Verification items for the finished model (mm, model axes). Face numbers are marked on the shaded views. Round coordinates to 2 decimals unless told otherwise and drop trailing zeros. Order: outer loops, then holes, each group sorted by start corner. A loop starts at its lowest first (then second) coordinate and runs counter-clockwise, first axis right, second up. Notation, with made-up numbers: M 66,32.5 L 121,32.5 A25 cw 121,46.5 Z; hole C -17,53.25 d1. An arc over 180 degrees is marked long. Use one line per item in the form item = value. Start each with the question number.
Item 1: Cross-section at B-B on x = -2.5. Count the separate pieces of the cut face and the enclosed holes in it, then the cut area to 3 significant figures.
Item 2: Go/stop test with a flat-tipped pin: pin 1 Ø2.5 at (y, z) = (-3.24, 4) entering from +X. Record where the tip stops, or that it passes through.
Item 3: Cross-section at A-A on z = 4. Enter the section's corners in (x, y), then the cut area to 3 significant figures.
Item 4: Thickness scan on probe 1 along Y at (x, z) = (3.25, 4); probe 2 along Y at (x, z) = (-6.5, 6.75); probe 3 along Y at (x, z) = (-1.75, 4). Record the ranges inside material, lowest first. Write a range as [from, to].
Item 5: Release check for a two-part mould opening along Y. For the marked faces 1, 2 and 3 record: +Y half, -Y half, draft (parallel to the pull), parting line (faces both ways), or undercut.
from build123d import *

# Parameters (mm, degrees)
EXTRUDE_1_DEPTH     = 8
SKETCH_2_R          = 1.7
CUT_EXTRUDE_2_DEPTH = 15
SKETCH_3_R          = 1.7
CUT_EXTRUDE_4_DEPTH = 15
CHAMFER_1_SIZE      = 0.5
SKETCH_4_R          = 1.7
CUT_EXTRUDE_5_DEPTH = 10


with BuildPart() as part:
    # 草图1 → 凸台-拉伸1 (new body)
    with BuildSketch(Plane.XY):
        with BuildLine():
            Line((-6.780789716, 23.005235362), (-6.780789716, 15.505235362))
            ThreePointArc((-6.780789716, 15.505235362), (0.719210284, 8.005235362), (-6.780789716, 0.505235362))
            Line((-6.780789716, 0.505235362), (-6.780789716, -6.994764638))
            ThreePointArc((-6.780789716, -6.994764638), (-0.358173427, -5.55020635), (4.82739705, -1.494764638))
            Line((4.82739705, -1.494764638), (4.82739705, 17.505235362))
            ThreePointArc((4.82739705, 17.505235362), (-0.358173427, 21.560677073), (-6.780789716, 23.005235362))
        make_face()
    extrude(amount=EXTRUDE_1_DEPTH)

    # 草图2 → 切除-拉伸2 (cut)
    with BuildSketch(Plane.ZY.offset(6.780789716)):
        with Locations((4, 19.255235362)):
            Circle(SKETCH_2_R)
    extrude(amount=-CUT_EXTRUDE_2_DEPTH, mode=Mode.SUBTRACT)

    # 草图3 → 切除-拉伸4 (cut)
    with BuildSketch(Plane.ZY.offset(6.780789716)):
        with Locations((4, -3.244764638)):
            Circle(SKETCH_3_R)
    extrude(amount=-CUT_EXTRUDE_4_DEPTH, mode=Mode.SUBTRACT)

    # 倒角1
    chamfer_1_edges = [part.edges().sort_by_distance(p)[0] for p in [
        (-0.358173427, -5.55020635, 8),
        (-0.358173427, 21.560677073, 8),
        (0.719210284, 8.005235362, 8),
        (-0.358173427, 21.560677073, 0),
        (-0.358173427, -5.55020635, 0),
        (0.719210284, 8.005235362, 0),
    ]]
    chamfer(chamfer_1_edges, length=CHAMFER_1_SIZE)

    # 草图4 → 切除-拉伸5 (cut)
    with BuildSketch(Plane(origin=(4.82739705, 0, 0), x_dir=(0, 0, -1), z_dir=(1, 0, 0))):
        with Locations((-4, 13.005235362)):
            Circle(SKETCH_4_R)
        with Locations((-4, 3.005235362)):
            Circle(SKETCH_4_R)
    extrude(amount=-CUT_EXTRUDE_5_DEPTH, mode=Mode.SUBTRACT)


solid = part.part
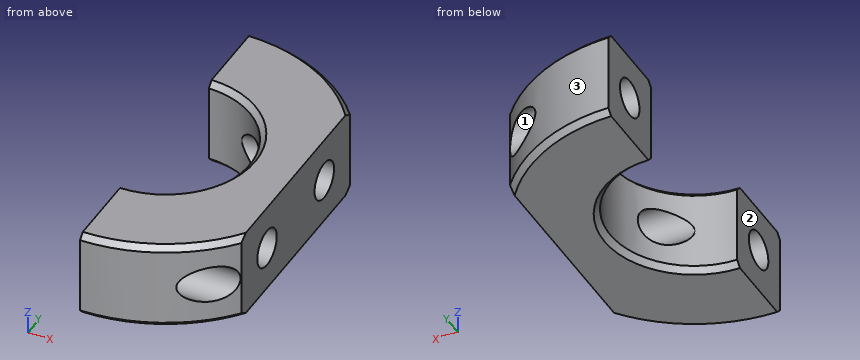
Output values:
q1.separate_pieces = 2
q1.enclosed_holes = 2
q1.area = 110 mm2
q2.pin_1 = through
q3.outline = M -6.78,-6.99 A15 ccw 0.79,-4.94 L -6.78,-4.94 Z; M -6.78,-1.54 L 4.79,-1.54 A15 ccw 4.83,-1.49 L 4.83,1.31 L -3.41,1.31 A7.5 cw -6.78,0.51 Z; M -6.78,15.51 A7.5 cw -3.41,14.71 L 4.83,14.71 L 4.83,17.51 A15 ccw 4.79,17.56 L -6.78,17.56 Z; M -6.78,20.96 L 0.79,20.96 A15 ccw -6.78,23.01 Z; M -0.05,4.71 L 4.83,4.71 L 4.83,11.31 L -0.05,11.31 A7.5 cw Z
q3.area = 112 mm2
q4.probe_1 = [-1.54, 1.31], [4.71, 11.31], [14.71, 17.56]
q4.probe_2 = [-6.99, 0.51], [15.5, 23]
q4.probe_3 = [-6.13, -4.94], [-1.54, 1.31], [14.71, 17.56], [20.96, 22.14]
q5.face_1 = undercut
q5.face_2 = draft
q5.face_3 = +Y half
